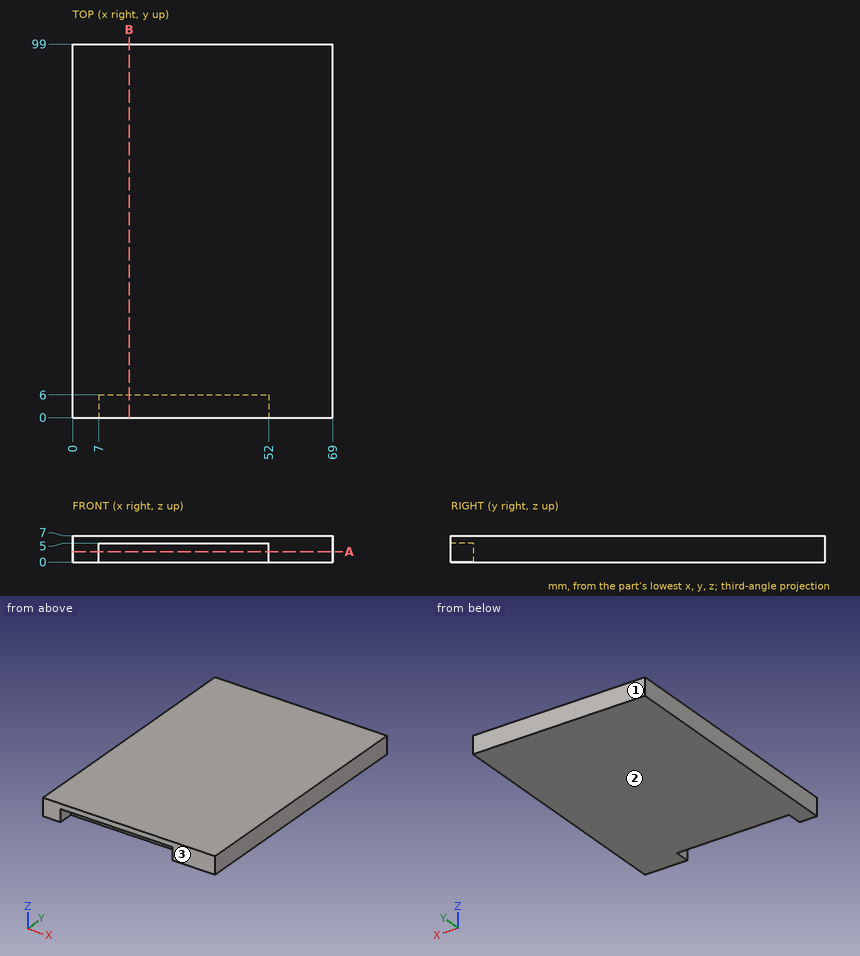
For this review, use the dimensioned drawing (mm, ordinates from the lowest corner) and the shaded views. Round coordinates to 2 decimals unless told otherwise and drop trailing zeros. Loops run counter-clockwise (first coordinate to the right, second up) from the corner with the lowest first, then second, coordinate; pieces in that order, holes last. Notation, with made-up numbers: M 39.5,-20.75 L 69.5,-20.75 A8 ccw 69.5,-15.75 Z; hole C -18,66.25 d5. An arc over 180 degrees is marked long. Answer as a JSON object with one key per item and string values.
(1) Take a section at A-A on z = 2.75. Give the boundary of the cut face in (x, y), and give its area (3 significant figures).
Resolved:
{"outline": "M 0,0 L 7,0 L 7,6 L 52,6 L 52,0 L 69,0 L 69,99 L 0,99 Z", "area": "6,560 mm²"}
(2) Draft analysis for pull direction Y (two halves, no side actions). For the marked faces 1, 2 and 3, state which applies: released by +Y, released by -Y, zero draft, split by the parting line, or undercut.
Resolved:
{"face 1": "released by +Y", "face 2": "zero draft", "face 3": "released by -Y"}
(3) Clearance check with flat-ended pins moving along their axes: P1, Ø6.5, axis at x = 25, y = 1.5, coming from the -Z side; P2, Ø4, axis at x = 38.5, z = 4.5, coming from the -Y side. State where each tip first meets the part, or that it passes through.
Resolved:
{"P1": "z = 5", "P2": "y = 0"}
(4) To check wall thickness, follow line 1 along Y through (x, z) = (51.5, 1). State the ranges of the line that lie inside material, in increasing order.
Resolved:
{"line 1": "6 to 99"}
(5) Take a section at B-B on x = 15. Give the boundary of the cut face in (y, z), and give its area (3 significant figures).
Resolved:
{"outline": "M 0,5 L 6,5 L 6,0 L 99,0 L 99,7 L 0,7 Z", "area": "663 mm²"}
